Can you work these out from the model? Positions are in its coordinate system, mm. Face numbers are marked on the shaded views. A direction names the side the tool comes from. Give positions to 0.01 mm unless a question says otherwise; leave off trailing zeros. Loops run counter-clockwise (first coordinate to the right, second up) from the corner with the lowest first, then second, coordinate; pieces in that order, holes last. Notation, with made-up numbers: (-31, 77) -> (-14, 77) arc R11 ccw to (-14, 96) -> close; hole circle Ø4 at (13.5, -11). An arc over 180 degrees is marked (long way). Return JSON: item names as keys, results as strings. Group by question number.
Q1. Will these pins go through, and if not, where does the flat tip stop? pin 1 (11 mm diameter, centred on x = -3, y = 11.5, fed in from +Z); pin 2 (4 mm diameter, centred on x = -2.5, z = 2.5, fed in from +Y); pin 3 (5 mm diameter, centred on x = -6, z = 4.5, fed in from -Y).
Q2. Suppose I cut it at D-D, the plane x = 8. Please give me the cut outline in (y, z).
Q3. Which directions (+Z, -Z, +X, -X, +Y, -Y) give clear straight access to the entire face, cutting with the end or side of a thin tool? Please do the marked faces 4, 5, 6, 7 and 8.
Q4. I need wall thicknesses on line 1 along X through (y, z) = (9.5, 6.25); line 2 along Z through (x, y) = (-13, 5); line 3 along X through (y, z) = (8.5, 8). Which ranges of each line are inside material? Lowest first, please. Write a range as [from, to].
Q5. Suppose I cut it at A-A, the plane y = 12.7. Count the separate pieces of the cut face and the enclosed holes in it, and give its area (3 significant figures).
Q6. Thinking about a two-plate mould opening in X: for the marked faces 1, 2 and 3, which applies, pulls with the +X half, pulls with the -X half, needs draft (parallel to the pull), parting line crosses it, or undercut?
Q7. Suppose I cut it at B-B, the plane z = 3.5. Please give me the cut outline in (x, y), and give its area (3 significant figures).
```python
from build123d import *

# Parameters (mm, degrees)
SKETCH1_R                 = 1.35255
BOSS_EXTRUDE1_DEPTH       = 25.4
SKETCH2_R                 = 3.937
CUT_EXTRUDE1_DEPTH        = 5.7625
M3X0_5_TAPPED_HOLE1_D     = 2.5
M3X0_5_TAPPED_HOLE1_DEPTH = 4.7625
CUT_EXTRUDE2_DEPTH        = 10.525


with BuildPart() as part:
    # Sketch1 → Boss-Extrude1 (new body)
    with BuildSketch(Plane(origin=(0, 0, 0), x_dir=(1, 0, 0), z_dir=(0, 1, 0))):
        Polygon((25.187315329, 0), (-25.187315329, 0), (-25.187315329, -9.525), (-20.711502729, -9.525), (-15.875, -4.7625), (15.875, -4.7625), (20.711502729, -9.525), (25.187315329, -9.525), align=None)
        with Locations((-22.012315329, -6.35)):
            Circle(SKETCH1_R, mode=Mode.SUBTRACT)
        with Locations((22.437684671, -6.35)):
            Circle(SKETCH1_R, mode=Mode.SUBTRACT)
    extrude(amount=BOSS_EXTRUDE1_DEPTH)

    # Sketch2 → Cut-Extrude1 (cut, through all)
    with BuildSketch(Plane.XY.offset(4.7625)):
        with Locations((-2.962315329, 12.7)):
            Circle(SKETCH2_R)
    extrude(amount=-CUT_EXTRUDE1_DEPTH, mode=Mode.SUBTRACT)

    # M3x0.5 Tapped Hole1
    with Locations(Plane.XY.offset(4.7625)):
        with Locations((7.537684671, 12.7)):
            Hole(M3X0_5_TAPPED_HOLE1_D / 2, depth=M3X0_5_TAPPED_HOLE1_DEPTH)

    # Sketch6 → Cut-Extrude2 (cut, through all)
    with BuildSketch(Plane(origin=(0, 0, 0), x_dir=(-1, 0, 0), z_dir=(0, 0, -1))):
        with BuildLine():
            Line((-17.4625, 25.4), (-12.972371939, 20.909871939))
            ThreePointArc((-12.972371939, 20.909871939), (-10.912283674, 19.533364969), (-8.482243879, 19.05))
            Line((-8.482243879, 19.05), (8.482243879, 19.05))
            ThreePointArc((8.482243879, 19.05), (10.912283674, 19.533364969), (12.972371939, 20.909871939))
            Line((12.972371939, 20.909871939), (17.4625, 25.4))
            Line((17.4625, 25.4), (-17.4625, 25.4))
        make_face()
        with BuildLine():
            Line((-17.4625, 0), (-12.972371939, 4.490128061))
            ThreePointArc((-12.972371939, 4.490128061), (-10.912283674, 5.866635031), (-8.482243879, 6.35))
            Line((-8.482243879, 6.35), (8.482243879, 6.35))
            ThreePointArc((8.482243879, 6.35), (10.912283674, 5.866635031), (12.972371939, 4.490128061))
            Line((12.972371939, 4.490128061), (17.4625, 0))
            Line((17.4625, 0), (-17.4625, 0))
        make_face()
    extrude(amount=-CUT_EXTRUDE2_DEPTH, mode=Mode.SUBTRACT)


solid = part.part
```
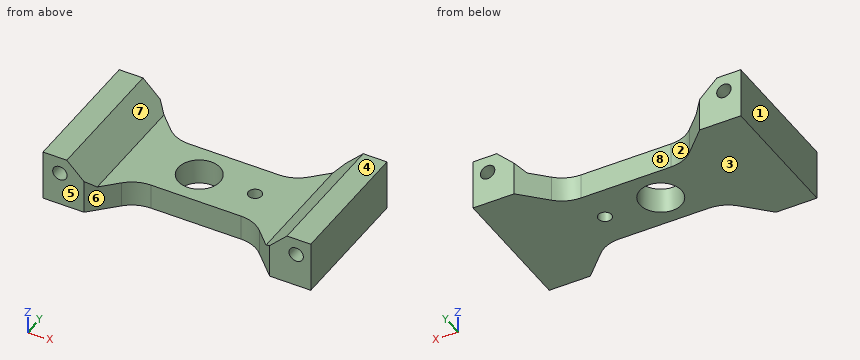
Ans:
{
 "1": {"pin 1": "stops at z = 4.76", "pin 2": "stops at y = 19.05", "pin 3": "stops at y = 6.35"},
 "2": {"outline": "(6.35, 0) -> (11.54, 0) -> (11.54, 4.76) -> (6.35, 4.76) -> close; (13.86, 0) -> (19.05, 0) -> (19.05, 4.76) -> (13.86, 4.76) -> close"},
 "3": {"face 4": "+Z, +X, -X, +Y, -Y", "face 5": "+Z, -Z, +X, -X, -Y", "face 6": "+Z, -Z, -Y", "face 7": "+Z, +Y, -Y", "face 8": "+Z, -Z, +Y"},
 "4": {"line 1": "x = [-25.19, -23.36], [-20.66, -17.39], [17.39, 21.09], [23.79, 25.19]", "line 2": "z = [0, 4.76]", "line 3": "x = [-25.19, -19.16], [19.16, 25.19]"},
 "5": {"separate pieces": "3", "enclosed holes": "2", "area": "245 mm^2"},
 "6": {"face 1": "pulls with the -X half", "face 2": "undercut", "face 3": "needs draft"},
 "7": {"outline": "(-25.19, 0) -> (-17.46, 0) -> (-12.97, 4.49) arc R6.35 cw to (-8.48, 6.35) -> (8.48, 6.35) arc R6.35 cw to (12.97, 4.49) -> (17.46, 0) -> (25.19, 0) -> (25.19, 25.4) -> (17.46, 25.4) -> (12.97, 20.91) arc R6.35 cw to (8.48, 19.05) -> (-8.48, 19.05) arc R6.35 cw to (-12.97, 20.91) -> (-17.46, 25.4) -> (-25.19, 25.4) -> close; hole circle Ø7.87 at (-2.96, 12.7); hole circle Ø2.5 at (7.54, 12.7)", "area": "866 mm^2"}
}
